Input: dimensioned drawing with shaded views. Units: mm. Origin: part minimum x, y, z. Give positions to 0.01 mm unless a question says otherwise; leave off trailing zeros. Loops run counter-clockwise (first coordinate to the right, second up) from the corner with the lowest first, then second, coordinate; pieces in that order, holes last. Notation, with made-up numbers: M 80.5,70.25 L 129.5,70.25 A14 cw 129.5,76.25 Z; hole C 65,65.5 d10. An arc over 180 degrees is marked long. Use CSV: the item, a comma, the result in double quotes. Start each with the question number.
Q1. Pull-direction query (X, two-part tool) for the marked faces 1, 2, 3 and 4; classes: released by +X, released by -X, zero draft, split by the parting line, or undercut.
Q2. Section B-B, the plane z = 3.5. Output: boundary loops of the cut face in (x, y) (3 decimals).
Q3. Section A-A, the plane y = 17.25. Output: boundary loops of the cut face in (x, z).
Q4. Material intervals for line 1 along X through (y, z) = (16.25, 1.5); line 2 along Z through (x, y) = (10.55, 26.5) (3 decimals); line 3 along X through (y, z) = (4, 3.5), sorted ascending.
Q5. Section C-C, the plane y = 26.5. Output: boundary loops of the cut face in (x, z) (3 decimals), plus the area to 3 significant figures.
Q6. Section D-D, the plane x = 6.05. Output: boundary loops of the cut face in (y, z), plus the area to 3 significant figures.
Q7. Pin query (flat end, axial travel): pin 1 (2 mm diameter, centred on x = 8, y = 10.5, fed in from -Z); pin 2 (3.5 mm diameter, centred on x = 5.5, z = 4.5, fed in from +Y); pin 3 (1.6 mm diameter, centred on x = 2, z = 1.5, fed in from -Y). Return the tip coordinate at first contact, or that it passes through.
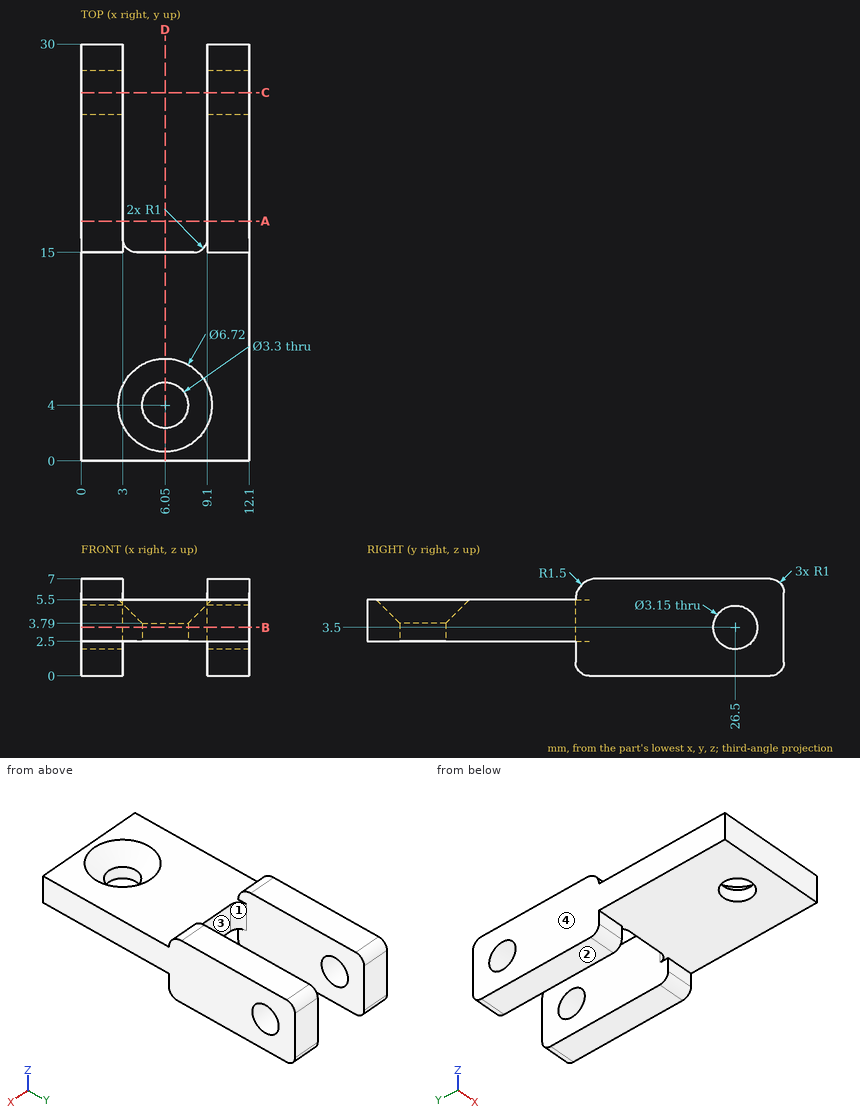
A:
1,face 1,"undercut"
1,face 2,"zero draft"
1,face 3,"undercut"
1,face 4,"released by -X"
2,outline,"M 0,0 L 12.1,0 L 12.1,24.925 L 9.1,24.925 L 9.1,16 A1 cw 8.1,15 L 4,15 A1 cw 3,16 L 3,24.925 L 0,24.925 Z; M 0,28.075 L 3,28.075 L 3,30 L 0,30 Z; M 9.1,28.075 L 12.1,28.075 L 12.1,30 L 9.1,30 Z; hole C 6.05,4 d3.3"
3,outline,"M 0,0 L 3,0 L 3,7 L 0,7 Z; M 9.1,0 L 12.1,0 L 12.1,7 L 9.1,7 Z"
4,line 1,"0 to 3, 9.1 to 12.1"
4,line 2,"0 to 1.925, 5.075 to 7"
4,line 3,"0 to 4.4, 7.7 to 12.1"
5,outline,"M 0,0 L 3,0 L 3,1.925 L 0,1.925 Z; M 0,5.075 L 3,5.075 L 3,7 L 0,7 Z; M 9.1,0 L 12.1,0 L 12.1,1.925 L 9.1,1.925 Z; M 9.1,5.075 L 12.1,5.075 L 12.1,7 L 9.1,7 Z"
5,area,"23.1 mm^2"
6,outline,"M 0,2.5 L 2.35,2.5 L 2.35,3.79 L 0.64,5.5 L 0,5.5 Z; M 5.65,2.5 L 15,2.5 L 15,5.5 L 7.36,5.5 L 5.65,3.79 Z"
6,area,"32.2 mm^2"
7,pin 1,"z = 2.5"
7,pin 2,"y = 15.03"
7,pin 3,"y = 15"
